Input: part model. Units: mm. Frame: model coordinates. A direction names the side the tool comes from. Coordinates: 2 decimals unless noted, no trailing zeros. Loops run counter-clockwise (first coordinate to the right, second up) from the corner with the lowest first, then second, coordinate; pieces in that order, holes last.
```python
from build123d import *

# Parameters (mm, degrees)
EXTRUDE_1_DEPTH     = 6
SKETCH_3_R          = 2.5
CUT_EXTRUDE_1_DEPTH = 13
FILLET_1_R          = 30
FILLET_2_R          = 1
SKETCH_6_R          = 1.5
CUT_EXTRUDE_3_DEPTH = 15
SKETCH_7_R          = 1.5
CUT_EXTRUDE_4_DEPTH = 15


with BuildPart() as part:
    # 草图1 → 凸台-拉伸1 (new body)
    with BuildSketch(Plane(origin=(0, 0, 0), x_dir=(1, 0, 0), z_dir=(0, 1, 0))):
        Polygon((-20, 60), (20, 60), (20, 11.547005384), (70, -17.320508076), (90, -28.867513459), (90, -78), (50, -78), (50, -51.961524227), (0, -23.094010768), (-50, -51.961524227), (-50, -78), (-90, -78), (-90, -28.867513459), (-70, -17.320508076), (-20, 11.547005384), align=None)
    extrude(amount=EXTRUDE_1_DEPTH)

    # 草图3 → 切除-拉伸1 (cut)
    with BuildSketch(Plane(origin=(0, 6, 0), x_dir=(1, 0, 0), z_dir=(0, 1, 0))):
        with Locations(Location((0, 37.498899984, 0), (0, 0, 270))):
            Circle(SKETCH_3_R)
        with Locations(Location((32.475, -18.749449992, 0), (0, 0, 270))):
            Circle(SKETCH_3_R)
        with Locations(Location((-32.475, -18.749449992, 0), (0, 0, 270))):
            Circle(SKETCH_3_R)
    extrude(amount=-CUT_EXTRUDE_1_DEPTH, mode=Mode.SUBTRACT)

    # 圆角1
    fillet_1_edges = [part.edges().sort_by_distance(p)[0] for p in [
        (-20, 3, -11.547005384),
        (20, 3, -11.547005384),
        (90, 3, 28.867513459),
        (50, 3, 51.961524227),
        (0, 3, 23.094010768),
        (-50, 3, 51.961524227),
        (-90, 3, 28.867513459),
    ]]
    fillet(fillet_1_edges, radius=FILLET_1_R)

    # 圆角2
    fillet_2_edges = [part.edges().sort_by_distance(p)[0] for p in [
        (-20, 3, -60),
        (20, 3, -60),
        (90, 3, 78),
        (50, 3, 78),
        (-50, 3, 78),
        (-90, 3, 78),
    ]]
    fillet(fillet_2_edges, radius=FILLET_2_R)

    # 草图6 → 切除-拉伸3 (cut)
    with BuildSketch(Plane.XY.offset(78)):
        with Locations((60, 3)):
            Circle(SKETCH_6_R)
        with Locations((85, 3)):
            Circle(SKETCH_6_R)
        with Locations(Location((-85, 3, 0), (0, 0, 180))):
            Circle(SKETCH_6_R)
        with Locations(Location((-60, 3, 0), (0, 0, 180))):
            Circle(SKETCH_6_R)
    extrude(amount=-CUT_EXTRUDE_3_DEPTH, mode=Mode.SUBTRACT)

    # 草图7 → 切除-拉伸4 (cut)
    with BuildSketch(Plane(origin=(0, 0, -60), x_dir=(-1, 0, 0), z_dir=(0, 0, -1))):
        with Locations((12.5, 3)):
            Circle(SKETCH_7_R)
        with Locations((-12.5, 3)):
            Circle(SKETCH_7_R)
    extrude(amount=-CUT_EXTRUDE_4_DEPTH, mode=Mode.SUBTRACT)


solid = part.part
```
Item 1: Line query: L1, parallel to Y at x = 85, z = 68; L2, parallel to Z at x = -0.5, y = 0.45; L3, parallel to X at y = 2.4, z = -27.5. Output: solid intervals per line, ascending.
Result:
L1: y = 0 to 1.5, 4.5 to 6
L2: z = -60 to -39.95, -35.05 to 27.74
L3: x = -20.03 to 20.03
Item 2: Section query A-A (x = 46). Output: boundary loops of the cut face in (y, z), then the cut area to 3 significant figures.
Result:
outline: (0, 3.46) - (6, 3.46) - (6, 54.32) - (0, 54.32) - close
area: 305 mm2
Item 3: Mould query, pull axis X, two halves, no side actions, for faces 1 (the face through (1, 0, 23)), 2 (the face through (46.09, 3.04, 54.47)), 3 (the face through (90, 3, 61)). Classes: +X half, -X half, draft (parallel to the pull), parting line (faces both ways), or undercut.
Result:
face 1: draft
face 2: undercut
face 3: +X half
Item 4: Section query C-C (y = 3). Count the separate pieces of the cut face and the enclosed holes in it, then the cut area to 3 significant figures.
Result:
separate pieces: 1
enclosed holes: 3
area: 11,000 mm2
Item 5: Contact query for flat-ended pins moving along their axis: P1, Ø1, axis at y = 3.5, z = 20, coming from the -X side; P2, Ø1.5, axis at x = -12, y = 3, coming from the -Z side; P3, Ø2.5, axis at x = -12.5, y = 3, coming from the +Z side; P4, Ø3.5, axis at x = 12.5, y = 3, coming from the -Z side. Output: stop coordinate, or through.
Result:
P1: stops at x = -75.5
P2: stops at z = -45
P3: stops at z = 31.07
P4: stops at z = -60
Item 6: Section query B-B (z = -8). Output: boundary loops of the cut face in (x, y).
Result:
outline: (-28.45, 0) - (28.45, 0) - (28.45, 6) - (-28.45, 6) - close
Item 7: Reachability of faces 4 (the face through (20, 3, -44)), 5 (the face through (-20, 3, -44)), 6 (the face through (-24.86, 2.958, 37.447)) from +Z, -Z, +X, -X, +Y, -Y: full face, straight path, thin tool, end or side. Return the list, or none.
Result:
face 4: -Z, +X, +Y, -Y
face 5: -Z, -X, +Y, -Y
face 6: +Z, +Y, -Y
